The model under review builds one solid part; all positions refer to its coordinate system, in mm. Give positions to 0.01 mm unless a question says otherwise; leave off trailing zeros. Loops run counter-clockwise (first coordinate to the right, second up) from the corner with the lowest first, then second, coordinate; pieces in that order, holes last. Notation, with made-up numbers: M 88.5,-15 L 125.5,-15 A35 ccw 125.5,19 Z; hole C 6,9.25 d9. An arc over 180 degrees is marked long. One line per item, written item: value. Start each with the question number.
Q1. To check wall thickness, follow line 1 along Y through (x, z) = (-6.5, 2.25); line 2 along X through (y, z) = (-16, 6.5); line 3 along Y through (x, z) = (0, 5.25). State the ranges of each line that lie inside material, in increasing order. Write a range as from..to.
Q2. For pin 1 (1 mm diameter, centred on x = -2.5, z = 1, fed in from +Y), flat-tipped, find the tip position at first contact; note if it passes through.
Q3. We need section A-A on x = 0. Write out the cut boundary in (y, z), plus the area to 3 significant figures.
Q4. We need section B-B on y = 5.5. Write out the cut boundary in (x, z), plus the area to 3 significant figures.
Q5. We need section C-C on x = -22. Write out the cut boundary in (y, z), plus the area to 3 significant figures.
Q6. We need section D-D on z = 1.75. Write out the cut boundary in (x, y) (3 decimals), plus the area to 3 significant figures.
Q7. Mouldability with a two-part tool opening along X and no side actions: class faces 1 (the face through (-42.67, -21.19, 3.76)), 2 (the face through (0, -12, 0)) as released by +X, released by -X, zero draft, split by the parting line, or undercut.
```python
from build123d import *

# Parameters (mm, degrees)
F0_R     = 11.0109
F1_DEPTH = 7.62


with BuildPart() as f1:
    # F0 (on Top) → F1 (new body)
    with BuildSketch(Plane.XY):
        with BuildLine():
            ThreePointArc((7.457027, 22.930229), (-2.538633, 20.940581), (-11.106239, 26.460369))
            ThreePointArc((-11.106239, 26.460369), (-11.625922, 8.457774), (-23.586674, -5.00714))
            ThreePointArc((-23.586674, -5.00714), (-18.127317, -10.016397), (-16.107352, -17.145))
            ThreePointArc((-16.107352, -17.145), (-16.42478, -20.064944), (-17.362233, -22.848469))
            ThreePointArc((-17.362233, -22.848469), (-1.511686, -14.29723), (16.129647, -17.923089))
            ThreePointArc((16.129647, -17.923089), (19.404391, -8.271769), (28.468471, -3.6119))
            ThreePointArc((28.468471, -3.6119), (13.137608, 5.839456), (7.457027, 22.930229))
        make_face()
        Circle(F0_R, mode=Mode.SUBTRACT)
        with BuildLine():
            ThreePointArc((43.28467, -17.145), (38.860372, -7.111748), (28.468471, -3.6119))
            ThreePointArc((28.468471, -3.6119), (19.404391, -8.271769), (16.129647, -17.923089))
            ThreePointArc((16.129647, -17.923089), (30.085215, -30.728084), (43.28467, -17.145))
        make_face()
        with Locations((29.696011, -17.145)):
            Circle(F0_R, mode=Mode.SUBTRACT)
        with BuildLine():
            ThreePointArc((-16.107352, -17.145), (-18.127317, -10.016397), (-23.586674, -5.00714))
            ThreePointArc((-23.586674, -5.00714), (-42.526264, -21.621189), (-17.362233, -22.848469))
            ThreePointArc((-17.362233, -22.848469), (-16.42478, -20.064944), (-16.107352, -17.145))
        make_face()
        with Locations((-29.696011, -17.145)):
            Circle(F0_R, mode=Mode.SUBTRACT)
        with BuildLine():
            ThreePointArc((7.457027, 22.930229), (11.957898, 27.835519), (13.588659, 34.29))
            ThreePointArc((13.588659, 34.29), (-4.10687, 47.243195), (-11.106239, 26.460369))
            ThreePointArc((-11.106239, 26.460369), (-2.538633, 20.940581), (7.457027, 22.930229))
        make_face()
        with Locations((0, 34.29)):
            Circle(F0_R, mode=Mode.SUBTRACT)
    extrude(amount=F1_DEPTH)


solid = f1.part
```
Solved:
1. line 1: -15.54..-8.89, 8.89..25.4, 43.18..46.22
1. line 2: -43.24..-40.65, -18.74..-7.71, 12.35..18.74, 40.65..43.24
1. line 3: -14.12..-11.01, 11.01..23.28, 45.3..47.88
2. pin 1: y = 47.73
3. outline: M -14.12,0 L -11.01,0 L -11.01,7.62 L -14.12,7.62 Z; M 11.01,0 L 23.28,0 L 23.28,7.62 L 11.01,7.62 Z; M 45.3,0 L 47.88,0 L 47.88,7.62 L 45.3,7.62 Z
3. area: 137 mm2
4. outline: M -13.02,0 L -9.54,0 L -9.54,7.62 L -13.02,7.62 Z; M 9.54,0 L 13.41,0 L 13.41,7.62 L 9.54,7.62 Z
4. area: 56.0 mm2
5. outline: M -28.34,0 L -25.02,0 L -25.02,7.62 L -28.34,7.62 Z; M -9.27,0 L -4.08,0 L -4.08,7.62 L -9.27,7.62 Z
5. area: 64.9 mm2
6. outline: M -23.587,-5.007 A13.589 ccw long -17.362,-22.848 A26.354 cw 16.13,-17.923 A13.589 ccw long 28.468,-3.612 A26.354 cw 7.457,22.93 A13.589 ccw long -11.106,26.46 A26.354 cw Z; hole C -29.696,-17.145 d22.022; hole C 0,0 d22.022; hole C 0,34.29 d22.022; hole C 29.696,-17.145 d22.022
6. area: 1,340 mm2
7. face 1: undercut
7. face 2: zero draft
